Check sheet for the modelled part. Datum: model origin and axes. Units: mm. Face numbers are marked on the shaded views. A direction names the side the tool comes from. Round coordinates to 2 decimals unless told otherwise and drop trailing zeros. Loops run counter-clockwise (first coordinate to the right, second up) from the corner with the lowest first, then second, coordinate; pieces in that order, holes last. Notation, with made-up numbers: (82, -23.5) - (108, -23.5) arc R6 ccw to (108, -17.5) - close; hole circle Ø2 at (35, 22). An arc over 180 degrees is marked (long way). Put each result on its own line as item: value. Start each with the question number.
Item 1: Gauge pin test, flat ends, axial feed: pin 1 Ø1.1 at (x, z) = (34, 14) entering from +Y; pin 2 Ø10 at (x, y) = (1.5, -3.5) entering from +Z; pin 3 Ø0.8 at (x, z) = (-28.5, 14) entering from -Y; pin 4 Ø5.5 at (x, y) = (0, 0) entering from -Z. Record the tip position at first contact, or that the pin passes through.
Item 2: Tool access check on the marked faces 1, 2 and 3. Record the directions out of +Z, -Z, +X, -X, +Y, -Y that give a thin tool (end or side, any length) a straight path to the whole face; none if there is none.
Item 3: Section check B-B, the plane x = -2. Record the cut outline in (y, z).
Item 4: Draft check along X on the marked faces 4, 5 and 6. Enter one of: pulls with the +X half, pulls with the -X half, needs draft (parallel to the pull), parting line crosses it, or undercut.
Item 5: Section check D-D, the plane x = -19. Record the cut outline in (y, z).
Item 6: Material ranges on line 1 along Y through (x, z) = (0, 3.75); line 2 along X through (y, z) = (0, 12.8); line 3 along Z through (x, y) = (-30, -0.75), recorded low to high.
Item 7: Section check A-A, the plane y = 0. Record the cut outline in (x, z), and give its area (3 significant figures).
Item 8: Section check C-C, the plane z = 7. Record the cut outline in (x, y).
from build123d import *

# Parameters (mm, degrees)
ESBO_O1_R                     = 5
ESBO_O1_R_2                   = 3.5
RESSALTO_EXTRUS_O1_DEPTH      = 10
ESBO_O2_R                     = 11
ESBO_O2_R_2                   = 3.5
RESSALTO_EXTRUS_O2_DEPTH      = 1
ESBO_O3_R                     = 11
ESBO_O3_R_2                   = 10
RESSALTO_EXTRUS_O3_DEPTH      = 3.5
CORTE_EXTRUS_O1_REACH         = 23.266
CORTE_EXTRUS_O1_END_RADIUS    = 11
ESBO_O4_W                     = 1.5
ESBO_O4_H                     = 3.5
RESSALTO_EXTRUS_O4_REACH      = 65.657
RESSALTO_EXTRUS_O4_END_RADIUS = 11
ESBO_O8_W                     = 1
ESBO_O8_H                     = 12


with BuildPart() as part:
    # Esboço1 → Ressalto-extrusão1 (new body)
    with BuildSketch(Plane.XY):
        Circle(ESBO_O1_R)
        Circle(ESBO_O1_R_2, mode=Mode.SUBTRACT)
    extrude(amount=RESSALTO_EXTRUS_O1_DEPTH)

    # Esboço2 → Ressalto-extrusão2 (add)
    with BuildSketch(Plane.XY.offset(10)):
        Circle(ESBO_O2_R)
        Circle(ESBO_O2_R_2, mode=Mode.SUBTRACT)
    extrude(amount=RESSALTO_EXTRUS_O2_DEPTH)

    # Esboço3 → Ressalto-extrusão3 (add)
    with BuildSketch(Plane.XY.offset(11)):
        Circle(ESBO_O3_R)
        Circle(ESBO_O3_R_2, mode=Mode.SUBTRACT)
    extrude(amount=RESSALTO_EXTRUS_O3_DEPTH)

    # Corte-extrusão1: up to this cylinder (the profile starts inside it)
    corte_extrus_o1_end = Plane(origin=(0, 0, 12.75), z_dir=(0, 0, -1)) * Cylinder(CORTE_EXTRUS_O1_END_RADIUS, 69.532, mode=Mode.PRIVATE)
    # Esboço4 → Corte-extrusão1 (cut, up to the surface)
    with BuildSketch(Plane(origin=(0, 0, 0), x_dir=(1, 0, 0), z_dir=(0, 1, 0)), mode=Mode.PRIVATE) as corte_extrus_o1_sk1:
        with Locations((0, -12.75)):
            Rectangle(ESBO_O4_W, ESBO_O4_H)
    corte_extrus_o1_tool1 = extrude(corte_extrus_o1_sk1.sketch, amount=-CORTE_EXTRUS_O1_REACH, mode=Mode.PRIVATE) & corte_extrus_o1_end
    add(corte_extrus_o1_tool1.solids().sort_by_distance((0, 0, 12.75))[0], mode=Mode.SUBTRACT)

    # Ressalto-extrusão4: up to this cylinder (the profile starts outside it)
    ressalto_extrus_o4_end = Plane(origin=(0, 0, 14), z_dir=(0, 0, -1)) * Cylinder(RESSALTO_EXTRUS_O4_END_RADIUS, 154.314, mode=Mode.PRIVATE)
    # Esboço8 → Ressalto-extrusão4 (add, up to the surface)
    with BuildSketch(Plane(origin=(50, 0, 0), x_dir=(0, 0, -1), z_dir=(1, 0, 0)), mode=Mode.PRIVATE) as ressalto_extrus_o4_sk1:
        with Locations((-14, -0.050414446)):
            Rectangle(ESBO_O8_W, ESBO_O8_H)
    ressalto_extrus_o4_tool1 = extrude(ressalto_extrus_o4_sk1.sketch, amount=-RESSALTO_EXTRUS_O4_REACH, mode=Mode.PRIVATE) - ressalto_extrus_o4_end
    ressalto_extrus_o4 = ressalto_extrus_o4_tool1.solids().sort_by_distance((50, -0.050414, 14))[0]
    add(ressalto_extrus_o4)

    # Espelhar1: Ressalto-extrusão4 across plane
    add(ressalto_extrus_o4.mirror(Plane(origin=(0, 0, 0), x_dir=(0, 0, 1), z_dir=(1, 0, 0))))


solid = part.part
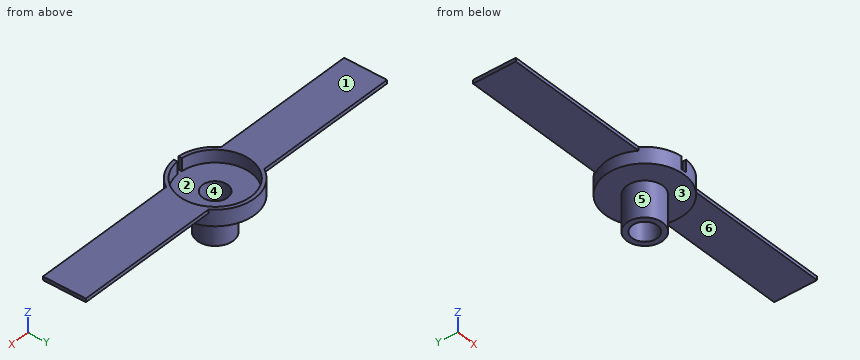
Check result:
1. pin 1: y = 5.95
1. pin 2: z = 11
1. pin 3: y = -6.05
1. pin 4: through
2. face 1: +Z, +X, -X, +Y, -Y
2. face 2: +Z
2. face 3: -Z
3. outline: (-10.82, 10) - (-4.58, 10) - (-4.58, 0) - (-2.87, 0) - (-2.87, 11) - (-9.8, 11) - (-9.8, 14.5) - (-10.82, 14.5) - close; (2.87, 0) - (4.58, 0) - (4.58, 10) - (10.82, 10) - (10.82, 14.5) - (9.8, 14.5) - (9.8, 11) - (2.87, 11) - close
4. face 4: undercut
4. face 5: parting line crosses it
4. face 6: needs draft
5. outline: (-6.05, 13.5) - (5.95, 13.5) - (5.95, 14.5) - (-6.05, 14.5) - close
6. line 1: -5 to -3.5, 3.5 to 5
6. line 2: -11 to -10, 10 to 11
6. line 3: 13.5 to 14.5
7. outline: (-50, 13.5) - (-11, 13.5) - (-11, 10) - (-5, 10) - (-5, 0) - (-3.5, 0) - (-3.5, 11) - (-10, 11) - (-10, 14.5) - (-50, 14.5) - close; (3.5, 0) - (5, 0) - (5, 10) - (11, 10) - (11, 13.5) - (50, 13.5) - (50, 14.5) - (10, 14.5) - (10, 11) - (3.5, 11) - close
7. area: 130 mm²
8. outline: circle Ø10 at (0, 0); hole circle Ø7 at (0, 0)
